from build123d import *

# Parameters (mm, degrees)
BASE_FLANGE1_DEPTH      = 3
F_10_CLEARANCE_HOLE1_D  = 5
EDGE_FLANGE1_DEPTH      = 112.7125
EDGE_FLANGE1_START      = 3
EDGE_FLANGE1_PROFILE_R  = 2.5
EDGE_FLANGE1_FLAT_DEPTH = 3


# Sheet-metal steps are written as plain solids
with BuildPart() as part:
    # Sketch7 → Base-Flange1 (new body)
    with BuildSketch(Plane(origin=(0, 0, 0), x_dir=(1, 0, 0), z_dir=(0, 1, 0))):
        Polygon((-56.35625, 15.875), (-56.35625, 3.6096), (56.35625, 3.6096), (56.35625, 15.875), (12.7, 69.85), (-12.7, 69.85), align=None)
    extrude(amount=-BASE_FLANGE1_DEPTH)

    # #10 Clearance Hole1 (through all)
    with Locations(Plane(origin=(0, -3, 0), x_dir=(-1, 0, 0), z_dir=(0, -1, 0))):
        with Locations((-50.8, 12.7), (50.8, 12.7), (-38.1, 25.4), (38.1, 25.4), (-25.4, 38.1), (-38.1, 12.7), (-25.4, 12.7), (-25.4, 25.4), (38.1, 12.7), (25.4, 12.7), (25.4, 38.1), (25.4, 25.4), (12.7, 38.1), (12.7, 25.4), (12.7, 12.7), (-12.7, 12.7), (-12.7, 25.4), (-12.7, 38.1), (-12.7, 50.8), (12.7, 50.8), (0, 63.5), (0, 50.8), (0, 38.1), (0, 25.4), (0, 12.7)):
            Hole(F_10_CLEARANCE_HOLE1_D / 2)

    # Edge-Flange1 bend section (across the edge) → Edge-Flange1 (add)
    with BuildSketch(Plane(origin=(56.35625, -3, -3), x_dir=(0, 0, -1), z_dir=(-1, 0, 0))):
        with BuildLine():
            Line((-3, 0.6096), (0, 0.6096))
            ThreePointArc((0, 0.6096), (0.178547706, 0.178547706), (0.6096, 0))
            Line((0.6096, 0), (0.6096, -3))
            ThreePointArc((0.6096, -3), (-1.942772637, -1.942772637), (-3, 0.6096))
        make_face()
    extrude(amount=EDGE_FLANGE1_DEPTH)

    # Edge-Flange1 profile (on flange) → Edge-Flange1 flat (add)
    with BuildSketch(Plane(origin=(0, -3, -3), x_dir=(-1, 0, 0), z_dir=(0, 0, 1)).offset(EDGE_FLANGE1_START)):
        Polygon((-56.35625, 0.6096), (56.35625, 0.6096), (56.35625, 12.875), (50.00625, 19.225), (-50.00625, 19.225), (-56.35625, 12.875), align=None)
        with Locations((50.8, 9.7)):
            Circle(EDGE_FLANGE1_PROFILE_R, mode=Mode.SUBTRACT)
        with Locations((38.1, 9.7)):
            Circle(EDGE_FLANGE1_PROFILE_R, mode=Mode.SUBTRACT)
        with Locations((25.4, 9.7)):
            Circle(EDGE_FLANGE1_PROFILE_R, mode=Mode.SUBTRACT)
        with Locations((12.7, 9.7)):
            Circle(EDGE_FLANGE1_PROFILE_R, mode=Mode.SUBTRACT)
        with Locations((0, 9.7)):
            Circle(EDGE_FLANGE1_PROFILE_R, mode=Mode.SUBTRACT)
        with Locations((-12.7, 9.7)):
            Circle(EDGE_FLANGE1_PROFILE_R, mode=Mode.SUBTRACT)
        with Locations((-25.4, 9.7)):
            Circle(EDGE_FLANGE1_PROFILE_R, mode=Mode.SUBTRACT)
        with Locations((-38.1, 9.7)):
            Circle(EDGE_FLANGE1_PROFILE_R, mode=Mode.SUBTRACT)
        with Locations((-50.8, 9.7)):
            Circle(EDGE_FLANGE1_PROFILE_R, mode=Mode.SUBTRACT)
    extrude(amount=-EDGE_FLANGE1_FLAT_DEPTH)


solid = part.part
Geometry check sheet. Reference: the model listing, model coordinates, mm. A direction names the side the tool comes from. Give positions to 0.01 mm unless a question says otherwise; leave off trailing zeros. Order: outer loops, then holes, each group sorted by start corner. A loop starts at its lowest first (then second) coordinate and runs counter-clockwise, first axis right, second up.
1) Tool access check on faces 1 (the cylindrical face through (-12.37, -15.18, -1.48)), 2 (the flat face through (-1, -3, -30)). Record the directions out of +Z, -Z, +X, -X, +Y, -Y that give a thin tool (end or side, any length) a straight path to the whole face; none if there is none.
Results are:
face 1: +Z, -Z
face 2: -Z, +X, -X, -Y
2) Cross-section at B-B (x = 4). Record the boundary of the cut face in (y, z) (3 decimals).
Results are:
outline: (-22.225, -3) - (-3.61, -3) arc R0.61 cw to (-3, -3.61) - (-3, -69.85) - (0, -69.85) - (0, -3.61) arc R3.61 ccw to (-3.61, 0) - (-22.225, 0) - close
3) Material ranges on probe 1 along Z at (x, y) = (-25.4, -0.65); probe 2 along Z at (x, y) = (-25.4, -1.3); probe 3 along Z at (x, y) = (12.7, -1.3), recorded low to high.
Results are:
probe 1: z = -54.15 to -40.6, -35.6 to -27.9, -22.9 to -15.2, -10.2 to -1.54
probe 2: z = -54.15 to -40.6, -35.6 to -27.9, -22.9 to -15.2, -10.2 to -0.84
probe 3: z = -69.85 to -53.3, -48.3 to -40.6, -35.6 to -27.9, -22.9 to -15.2, -10.2 to -0.84
4) Cross-section at C-C (z = -38.1). Record the boundary of the cut face in (x, y).
Results are:
outline: (-38.38, -3) - (-27.9, -3) - (-27.9, 0) - (-38.38, 0) - close; (-22.9, -3) - (-15.2, -3) - (-15.2, 0) - (-22.9, 0) - close; (-10.2, -3) - (-2.5, -3) - (-2.5, 0) - (-10.2, 0) - close; (2.5, -3) - (10.2, -3) - (10.2, 0) - (2.5, 0) - close; (15.2, -3) - (22.9, -3) - (22.9, 0) - (15.2, 0) - close; (27.9, -3) - (38.38, -3) - (38.38, 0) - (27.9, 0) - close
5) Gauge pin test, flat ends, axial feed: pin 1 (8 mm diameter, centred on x = 39, y = -18, fed in from -Z); pin 2 (4 mm diameter, centred on x = -38.1, z = -25.4, fed in from -Y); pin 3 (5 mm diameter, centred on x = -31.5, z = -43, fed in from -Y); pin 4 (8 mm diameter, centred on x = 12.7, y = -12.7, fed in from +Z). Record the tip position at first contact, or that the pin passes through.
Results are:
pin 1: stops at z = -3
pin 2: passes through
pin 3: stops at y = -3
pin 4: stops at z = 0
6) Cross-section at A-A (z = -50.8). Record the boundary of the cut face in (x, y), then the cut area to 3 significant figures.
Results are:
outline: (-28.11, -3) - (-15.2, -3) - (-15.2, 0) - (-28.11, 0) - close; (-10.2, -3) - (-2.5, -3) - (-2.5, 0) - (-10.2, 0) - close; (2.5, -3) - (10.2, -3) - (10.2, 0) - (2.5, 0) - close; (15.2, -3) - (28.11, -3) - (28.11, 0) - (15.2, 0) - close
area: 124 mm2
7) Cross-section at D-D (x = -39). Record the boundary of the cut face in (y, z) (3 decimals), then the cut area to 3 significant figures.
Results are:
outline: (-22.225, -3) - (-15.032, -3) - (-15.032, 0) - (-22.225, 0) - close; (-10.368, -3) - (-3.61, -3) arc R0.61 cw to (-3, -3.61) - (-3, -10.368) - (0, -10.368) - (0, -3.61) arc R3.61 ccw to (-3.61, 0) - (-10.368, 0) - close; (-3, -37.334) - (0, -37.334) - (0, -27.732) - (-3, -27.732) - close; (-3, -23.068) - (0, -23.068) - (0, -15.032) - (-3, -15.032) - close
area: 125 mm2
8) Draft check along Y on faces 3 (the cylindrical face through (53.3, -12.8, -1.5)), 4 (the cylindrical face through (-35.715, -1.479, -26.151)), 5 (the cylindrical face through (0.789, -1.029, -1.085)). Enter one of: released by +Y, released by -Y, zero draft, split by the parting line, or undercut.
Results are:
face 3: undercut
face 4: zero draft
face 5: released by +Y
